Build history of the part. All positions in model axes, mm. Face numbers are marked on the shaded views. A direction names the side the tool comes from. Coordinates: 2 decimals unless noted, no trailing zeros. Loops run counter-clockwise (first coordinate to the right, second up) from the corner with the lowest first, then second, coordinate; pieces in that order, holes last.
(1) Tool access for the marked faces 4 and 5: list every direction of +Z, -Z, +X, -X, +Y, -Y with a clear straight run to the whole face (end or side of a thin tool).
(2) Flat gauge pins, fed straight in: P1, Ø6.5, axis at x = 49, y = 0, coming from the -Z side; P2, Ø0.7, axis at y = -18, z = 1, coming from the -X side; P3, Ø5, axis at x = -49, y = 0, coming from the +Z side; P4, Ø2.5, axis at y = -15.5, z = 1.5, coming from the -X side. Where does each tip first touch, or does it go through?
(3) Two-plate mould, pull along Y, no slides. Class the marked faces 1, 2 and 3: pulls with the +Y half, pulls with the -Y half, needs draft (parallel to the pull), parting line crosses it, or undercut.
(4) Slice it at B-B (y = 0). Give the cut face in (x, z).
(5) Wall check: L1, parallel to X at y = 6, z = 1.5; L2, parallel to X at y = 0, z = -1.55; L3, parallel to Y at x = 23, z = 1.25. Give the ranges that are in metal, low to high.
(6) Slice it at C-C (x = 15). Give the cut face in (y, z), and give its area (3 significant figures).
(7) Slice it at A-A (x = 3). Give the cut face in (y, z), and give its area (3 significant figures).
(8) Slice it at D-D (y = -24.5). Give the cut face in (x, z), and give its area (3 significant figures).
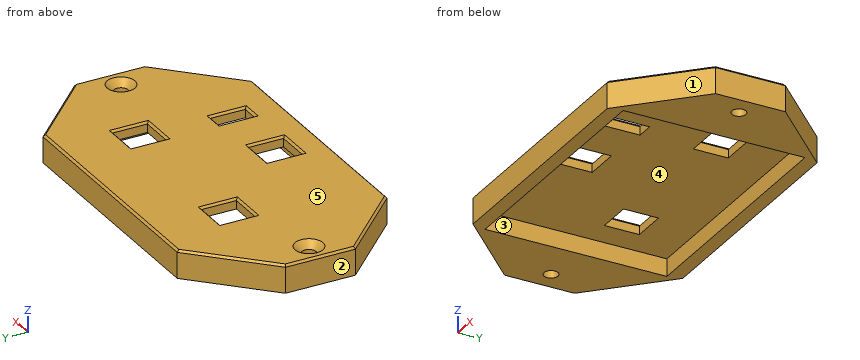
Autodesk Inventor part; units mm, degrees
ref_plane "YZ Plane" through (0, 0, 0) normal (1, 0, 0) x (0, 1, 0)
ref_plane "XZ Plane" through (0, 0, 0) normal (0, 1, 0) x (-1, 0, 0)
ref_plane "XY Plane" through (0, 0, 0) normal (0, 0, 1) x (1, 0, 0)
sketch "Sketch1" plane through (0, 0, 0) normal (0, 0, 1) x (1, 0, 0)
  line L0 (-28, 3.75) -> (-18, 3.75)
  line L1 (-18, 3.75) -> (-18, 13.75)
  line L2 (-18, 13.75) -> (-28, 13.75)
  line L3 (-28, 13.75) -> (-28, 3.75)
  line L4 (-28, 3.75) -> (-18, 13.75) construction
  line L5 (-18, 3.75) -> (-28, 13.75) construction
  line L6 (18.38, 3.75) -> (28.38, 3.75)
  line L7 (28.38, 3.75) -> (28.38, 13.75)
  line L8 (28.38, 13.75) -> (18.38, 13.75)
  line L9 (18.38, 13.75) -> (18.38, 3.75)
  line L10 (18.38, 3.75) -> (28.38, 13.75) construction
  line L11 (28.38, 3.75) -> (18.38, 13.75) construction
  line L12 (-4.75, -12.5) -> (5.25, -12.5)
  line L13 (5.25, -12.5) -> (5.25, -22.5)
  line L14 (5.25, -22.5) -> (-4.75, -22.5)
  line L15 (-4.75, -22.5) -> (-4.75, -12.5)
  line L16 (-4.75, -12.5) -> (5.25, -22.5) construction
  line L17 (5.25, -12.5) -> (-4.75, -22.5) construction
  circle A0 centre (-23, 8.75) radius 1.925 construction
  circle A1 centre (23.38, 8.75) radius 1.925 construction
  circle A2 centre (0.25, -17.5) radius 1.925 construction
  line L18 (21.5954, -14.7725) -> (21.5954, -18.3725) construction
  line L19 (19.9954, -14.7725) -> (21.5954, -14.7725) construction
  line L20 (19.9954, -18.3725) -> (19.9954, -14.7725) construction
  line L21 (21.5954, -18.3725) -> (19.9954, -18.3725) construction
  line L22 (21.5454, -18.3225) -> (20.0454, -18.3225) construction
  line L23 (20.0454, -18.3225) -> (20.0454, -16.8225) construction
  line L24 (20.0454, -16.8225) -> (21.5454, -16.8225) construction
  line L25 (21.5454, -16.8225) -> (21.5454, -18.3225) construction
  line L26 (18.4, -21.5) -> (23.4, -21.5)
  line L27 (23.4, -21.5) -> (23.4, -11.5)
  line L28 (23.4, -11.5) -> (18.4, -11.5)
  line L29 (18.4, -11.5) -> (18.4, -21.5)
  line L30 (18.4, -21.5) -> (23.4, -11.5) construction
  line L31 (23.4, -21.5) -> (18.4, -11.5) construction
  circle A3 centre (22.55, -16.5) radius 0.45 construction
  circle A4 centre (19.25, -16.5) radius 0.45 construction
  line L32 (19.25, -16.5) -> (22.55, -16.5) construction
  line L33 (-45, -30) -> (45, -30)
  line L34 (45, -30) -> (45, 30)
  line L35 (45, 30) -> (-45, 30)
  line L36 (-45, 30) -> (-45, -30)
  line L37 (-45, -30) -> (45, 30) construction
  line L38 (45, -30) -> (-45, 30) construction
  line L39 (-30, 25) -> (30, 25)
  line L40 (35, 20) -> (35, -20)
  point P0 (0, 0)
  point P1 (23.38, 8.75)
  point P2 (0.25, -17.5)
  point P3 (20.9, -16.5)
  point P4 (20.9, -16.5)
  dimension "d0" = 10
  dimension "d3" = 5
  dimension "d4" = 10
  dimension "d5" = 10
  dimension "d6" = 5
extrude "Extrusion1" add sketch "Sketch1" along normal blind 3
sketch "Sketch2" plane through (0, 0, 0) normal (0, 0, -1) x (-1, 0, 0)
  line L0 (36, 26) -> (-36, 26)
  line L1 (-36, 26) -> (-36, -26)
  line L2 (-36, -26) -> (36, -26)
  line L3 (36, -26) -> (36, 26)
  line L4 (36, 26) -> (-36, -26) construction
  line L5 (-36, 26) -> (36, -26) construction
  line L6 (-30, -25) -> (30, -25)
  line L7 (35, -20) -> (35, 20)
  line L8 (-45, -30) -> (-45, 30)
  line L9 (45, -30) -> (-45, -30)
  line L10 (45, 30) -> (45, -30)
  line L11 (-45, 30) -> (45, 30)
  line L12 (-18.4, -21.5) -> (-18.4, -11.5)
  line L13 (-23.4, -21.5) -> (-18.4, -21.5)
  line L14 (-23.4, -11.5) -> (-23.4, -21.5)
  line L15 (-18.4, -11.5) -> (-23.4, -11.5)
  line L16 (4.75, -12.5) -> (-5.25, -12.5)
  line L17 (4.75, -22.5) -> (4.75, -12.5)
  line L18 (-5.25, -22.5) -> (4.75, -22.5)
  line L19 (-5.25, -12.5) -> (-5.25, -22.5)
  line L20 (-18.38, 3.75) -> (-18.38, 13.75)
  line L21 (-28.38, 3.75) -> (-18.38, 3.75)
  line L22 (-28.38, 13.75) -> (-28.38, 3.75)
  line L23 (-18.38, 13.75) -> (-28.38, 13.75)
  line L24 (28, 3.75) -> (28, 13.75)
  line L25 (18, 3.75) -> (28, 3.75)
  line L26 (18, 13.75) -> (18, 3.75)
  line L27 (28, 13.75) -> (18, 13.75)
  point P0 (0, 0)
  dimension "d9" = 1
  dimension "d10" = 1
extrude "Extrusion2" add sketch "Sketch2" along normal blind 5 contours L8 L11 L10 L9
chamfer "Chamfer1" distance 10 angle 45 4 edges at (-45, -30, -1) (45, -30, -1) (45, 30, -1) (-45, 30, -1)
sketch "Sketch3" plane through (0, 0, 3) normal (0, 0, 1) x (1, 0, 0)
  line L0 (45, -20) -> (45, 20)
  line L1 (45, -20) -> (55, -10)
  line L2 (55, -10) -> (55, 10)
  line L3 (55, 10) -> (45, 20)
  line L4 (45, -20) -> (35, -30)
  line L5 (35, 30) -> (45, 20)
  line L6 (-65, 0) -> (75, 0) construction
  point P0 (0, 0)
  point P1 (49, 0)
  dimension "d16" = 10
  dimension "d17" = 6
extrude "Extrusion3" add sketch "Sketch3" against normal up to surface (8 mm away)
hole "Hole1" at (49, 0, 3) direction (0, 0, -1) diameter 4 end through all countersink diameter 8 countersink angle 90
mirror "Mirror1" about plane through (0, 0, 0) normal (1, 0, 0) of "Extrusion3", "Hole1"
chamfer "Chamfer2" distance 0.6 angle 45 24 edges at (45, -20, 3) (55, 0, 3) (45, 20, 3) (0, 30, 3) (-45, 20, 3) (-55, 0, 3) (-45, -20, 3) (0, -30, 3) (-28, 8.75, 3) (-23, 3.75, 3) (-18, 8.75, 3) (-23, 13.75, 3) (23.38, 13.75, 3) (28.38, 8.75, 3) (23.38, 3.75, 3) (18.38, 8.75, 3) (20.9, -11.5, 3) (18.4, -16.5, 3) (20.9, -21.5, 3) (23.4, -16.5, 3) (5.25, -17.5, 3) (0.25, -22.5, 3) (-4.75, -17.5, 3) (0.25, -12.5, 3)
properties part number "_3DPrint"
Response values:
1. face 4: -Z
1. face 5: +Z, +X, -X, +Y, -Y
2. P1: stops at z = -5
2. P2: stops at x = -47.35
2. P3: stops at z = 1.5
2. P4: stops at x = -50.75
3. face 1: pulls with the -Y half
3. face 2: needs draft
3. face 3: undercut
4. outline: (-55, -5) - (-51, -5) - (-51, 1) - (-53, 3) - (-54.4, 3) - (-55, 2.4) - close; (-47, -5) - (-36, -5) - (-36, 0) - (36, 0) - (36, -5) - (47, -5) - (47, 1) - (45, 3) - (-45, 3) - (-47, 1) - close; (51, -5) - (55, -5) - (55, 2.4) - (54.4, 3) - (53, 3) - (51, 1) - close
5. L1: x = -55 to -28, -18 to 18.38, 28.38 to 55
5. L2: x = -55 to -51, -47 to -36, 36 to 47, 51 to 55
5. L3: y = -30 to -21.5, -11.5 to 3.75, 13.75 to 30
6. outline: (-30, -5) - (-26, -5) - (-26, 0) - (26, 0) - (26, -5) - (30, -5) - (30, 2.4) - (29.4, 3) - (-29.4, 3) - (-30, 2.4) - close
6. area: 220 mm2
7. outline: (-30, -5) - (-26, -5) - (-26, 0) - (-22.5, 0) - (-22.5, 2.4) - (-23.1, 3) - (-29.4, 3) - (-30, 2.4) - close; (-12.5, 0) - (26, 0) - (26, -5) - (30, -5) - (30, 2.4) - (29.4, 3) - (-11.9, 3) - (-12.5, 2.4) - close
7. area: 189 mm2
8. outline: (-40.5, -5) - (-36, -5) - (-36, 0) - (36, 0) - (36, -5) - (40.5, -5) - (40.5, 2.4) - (39.65, 3) - (-39.65, 3) - (-40.5, 2.4) - close
8. area: 287 mm2
